Source: CAD feature listing. Evaluate the final solid. Frame: model axes, mm. Face numbers are marked on the shaded views. A direction names the side the tool comes from. Coordinates: 2 decimals unless noted, no trailing zeros. Loops run counter-clockwise (first coordinate to the right, second up) from the corner with the lowest first, then second, coordinate; pieces in that order, holes last.
Item 1: Section query D-D, the plane x = 27. Return the cut outline in (y, z).
Item 2: Reachability of the marked faces 5, 6 and 7 from +Z, -Z, +X, -X, +Y, -Y: full face, straight path, thin tool, end or side. Return the list, or none.
Item 3: Section query A-A, the plane y = 0. Return the cut outline in (x, z), then the cut area to 3 significant figures.
Item 4: Pull-direction query (Y, two-part tool) for the marked faces 1, 2, 3 and 4; classes: +Y half, -Y half, draft (parallel to the pull), parting line (faces both ways), or undercut.
Item 5: Line query: probe 1 along Y at (x, z) = (32.5, 0.75); probe 2 along X at (y, z) = (2.5, -3). Output: solid intervals per line, ascending.
Item 6: Section query B-B, the plane z = -14.5. Return the cut outline in (x, y), then the cut area to 3 significant figures.
Item 7: Pin query (flat end, axial travel): pin 1 Ø7 at (y, z) = (1, -4) entering from +X; pin 2 Ø10 at (y, z) = (13, -9.5) entering from -X; pin 3 Ø2 at (y, z) = (-11, -13) entering from +X; pin 4 Ø10 at (y, z) = (2.5, -2) entering from -X. Return the tip coordinate at first contact, or that it passes through.
Item 8: Section query C-C, the plane y = 10. Return the cut outline in (x, z).
```python
from build123d import *

# Parameters (mm, degrees)
F0_W             = 75
F0_H             = 35
F1_DEPTH         = 1
F3_DEPTH         = 30
F5_DEPTH         = 35
F6_R             = 5
F7_R             = 1.75
F8_DEPTH         = 25
F9_DEPTH         = 1
F10_DEPTH        = 65.4
F13_DEPTH        = 35.6
F13_COPIES_COUNT = 6
F14_T1_DEPTH     = 16.1153550717
F14_T3_DEPTH     = 16.1153550717
F14_T5_DEPTH     = 16.1153550717
F14_T7_DEPTH     = 16.1153550717
F14_T9_DEPTH     = 16.1153550717
F14_T11_DEPTH    = 16.1153550717
F14_T13_DEPTH    = 16.1153550717
F14_T15_DEPTH    = 16.1153550717
F14_T17_DEPTH    = 16.1153550717
F14_T19_DEPTH    = 16.1153550717


# Not quite as in the source:
# - a fillet or chamfer that OpenCascade refuses, or shapes differently, is made with other operations: its cross-section is extruded or revolved along the edge and cut away or added
# - a pattern or mirror of a feature is missing from the dataset's text; its kind, count and spacing are read off the source's solid


with BuildPart() as f1:
    # F0 (on Top) → F1 (new body)
    with BuildSketch(Plane.XY):
        Rectangle(F0_W, F0_H)
    extrude(amount=F1_DEPTH)

    # F2 (on Top) → F3 (join)
    with BuildSketch(Plane.XY):
        Polygon((24.1481456572, 6.4704761276), (17.6776695297, 17.6776695297), (6.4704761276, 24.1481456572), (-6.4704761276, 24.1481456572), (-17.6776695297, 17.6776695297), (-24.1481456572, 6.4704761276), (-24.1481456572, -6.4704761276), (-17.6776695297, -17.6776695297), (-6.4704761276, -24.1481456572), (6.4704761276, -24.1481456572), (17.6776695297, -17.6776695297), (24.1481456572, -6.4704761276), align=None)
    extrude(amount=-F3_DEPTH)

    # F4 (on face) → F5 (cut)
    with BuildSketch(Plane(origin=(0, 0, -30), x_dir=(1, 0, 0), z_dir=(0, 0, -1))):
        Polygon((6.2116570825, -23.1822198309), (16.9705627485, -16.9705627485), (23.1822198309, -6.2116570825), (23.1822198309, 6.2116570825), (16.9705627485, 16.9705627485), (6.2116570825, 23.1822198309), (-6.2116570825, 23.1822198309), (-16.9705627485, 16.9705627485), (-23.1822198309, 6.2116570825), (-23.1822198309, -6.2116570825), (-16.9705627485, -16.9705627485), (-6.2116570825, -23.1822198309), align=None)
    extrude(amount=-F5_DEPTH, mode=Mode.SUBTRACT)

    # F6
    f6_edges = [f1.edges().sort_by_distance(p)[0] for p in [
        (37.5, -17.5, 0.5),
        (37.5, 17.5, 0.5),
        (-37.5, -17.5, 0.5),
        (-37.5, 17.5, 0.5),
    ]]
    fillet(f6_edges, radius=F6_R)

    # F7 (on Top) → F8 (cut)
    with BuildSketch(Plane.XY):
        with Locations((-32.5, 10)):
            Circle(F7_R)
        with Locations((-32.5, -10)):
            Circle(F7_R)
        with Locations((32.5, -10)):
            Circle(F7_R)
        with Locations((32.5, 10)):
            Circle(F7_R)
    extrude(amount=F8_DEPTH, mode=Mode.SUBTRACT)

    # F2 (on Top) → F9 (join)
    with BuildSketch(Plane.XY):
        Polygon((24.1481456572, 6.4704761276), (17.6776695297, 17.6776695297), (6.4704761276, 24.1481456572), (-6.4704761276, 24.1481456572), (-17.6776695297, 17.6776695297), (-24.1481456572, 6.4704761276), (-24.1481456572, -6.4704761276), (-17.6776695297, -17.6776695297), (-6.4704761276, -24.1481456572), (6.4704761276, -24.1481456572), (17.6776695297, -17.6776695297), (24.1481456572, -6.4704761276), align=None)
    extrude(amount=F9_DEPTH)

    # F4 (on face) → F10 (cut)
    with BuildSketch(Plane(origin=(0, 0, -30), x_dir=(1, 0, 0), z_dir=(0, 0, -1))):
        Polygon((6.2116570825, -23.1822198309), (16.9705627485, -16.9705627485), (23.1822198309, -6.2116570825), (23.1822198309, 6.2116570825), (16.9705627485, 16.9705627485), (6.2116570825, 23.1822198309), (-6.2116570825, 23.1822198309), (-16.9705627485, 16.9705627485), (-23.1822198309, 6.2116570825), (-23.1822198309, -6.2116570825), (-16.9705627485, -16.9705627485), (-6.2116570825, -23.1822198309), align=None)
    extrude(amount=-F10_DEPTH, mode=Mode.SUBTRACT)

    # F12 (on Right) → F13 (cut)
    with BuildSketch(Plane.YZ):
        with BuildLine():
            ThreePointArc((-8, -13), (0, -21), (8, -13))
            ThreePointArc((8, -13), (0, -5), (-8, -13))
        make_face()
        with BuildLine():
            Line((8, -37.0977148414), (8, -13))
            ThreePointArc((8, -13), (0, -21), (-8, -13))
            Line((-8, -13), (-8, -36.2910553813))
            Line((-8, -36.2910553813), (8, -37.0977148414))
        make_face()
    f13 = extrude(amount=F13_DEPTH, mode=Mode.SUBTRACT)

    # F13_copies: F13 ×6 about axis
    f13_copies_axis = Axis((0, 0, 0), (0, 0, 1))
    for i in range(1, F13_COPIES_COUNT):
        add(f13.rotate(f13_copies_axis, i * 360 / F13_COPIES_COUNT), mode=Mode.SUBTRACT)

    # F14: fillet of radius 3 on 12 edges, made by hand

    # F14_s2 → F14_t1 (cut)
    with BuildSketch(Plane.YZ.offset(14.6497195661)):
        with BuildLine():
            ThreePointArc((-11, -30), (-8.8786796564, -29.1213203436), (-8, -27))
            Line((-8, -27), (-8, -30))
            Line((-8, -30), (-11, -30))
        make_face()
        with BuildLine():
            ThreePointArc((8, -27), (8.8786796564, -29.1213203436), (11, -30))
            Line((11, -30), (8, -30))
            Line((8, -30), (8, -27))
        make_face()
    extrude(amount=F14_T1_DEPTH, mode=Mode.SUBTRACT)

    # F14_s4 → F14_t3 (cut)
    with BuildSketch(Plane.YZ.offset(-30.7650746377)):
        with BuildLine():
            ThreePointArc((-8, -27), (-8.8786796564, -29.1213203436), (-11, -30))
            Line((-11, -30), (-8, -30))
            Line((-8, -30), (-8, -27))
        make_face()
        with BuildLine():
            ThreePointArc((8, -27), (8.8786796564, -29.1213203436), (11, -30))
            Line((11, -30), (8, -30))
            Line((8, -30), (8, -27))
        make_face()
    extrude(amount=F14_T3_DEPTH, mode=Mode.SUBTRACT)

    # F14_s6 → F14_t5 (cut)
    with BuildSketch(Plane(origin=(-15.3825373189, -26.6433361856, 0), x_dir=(0, 0, 1), z_dir=(0.5, 0.8660254038, 0))):
        with BuildLine():
            ThreePointArc((-30, -11), (-29.1213203436, -8.8786796564), (-27, -8))
            Line((-27, -8), (-30, -8))
            Line((-30, -8), (-30, -11))
        make_face()
    extrude(amount=F14_T5_DEPTH, mode=Mode.SUBTRACT)

    # F14_s8 → F14_t7 (cut)
    with BuildSketch(Plane(origin=(-7.324859783, 12.6870293026, 0), x_dir=(0, 0, 1), z_dir=(-0.5, 0.8660254038, 0))):
        with BuildLine():
            ThreePointArc((-30, -11), (-29.1213203436, -8.8786796564), (-27, -8))
            Line((-27, -8), (-30, -8))
            Line((-30, -8), (-30, -11))
        make_face()
    extrude(amount=F14_T7_DEPTH, mode=Mode.SUBTRACT)

    # F14_s10 → F14_t9 (cut)
    with BuildSketch(Plane(origin=(-7.324859783, -12.6870293026, 0), x_dir=(0, 0, 1), z_dir=(-0.5, -0.8660254038, 0))):
        with BuildLine():
            ThreePointArc((-27, -8), (-29.1213203436, -8.8786796564), (-30, -11))
            Line((-30, -11), (-30, -8))
            Line((-30, -8), (-27, -8))
        make_face()
    extrude(amount=F14_T9_DEPTH, mode=Mode.SUBTRACT)

    # F14_s12 → F14_t11 (cut)
    with BuildSketch(Plane(origin=(7.324859783, 12.6870293026, 0), x_dir=(0, 0, 1), z_dir=(0.5, 0.8660254038, 0))):
        with BuildLine():
            ThreePointArc((-27, -8), (-29.1213203436, -8.8786796564), (-30, -11))
            Line((-30, -11), (-30, -8))
            Line((-30, -8), (-27, -8))
        make_face()
    extrude(amount=F14_T11_DEPTH, mode=Mode.SUBTRACT)

    # F14_s14 → F14_t13 (cut)
    with BuildSketch(Plane(origin=(-15.3825373189, 26.6433361856, 0), x_dir=(0, 0, 1), z_dir=(0.5, -0.8660254038, 0))):
        with BuildLine():
            ThreePointArc((-30, -11), (-29.1213203436, -8.8786796564), (-27, -8))
            Line((-27, -8), (-30, -8))
            Line((-30, -8), (-30, -11))
        make_face()
    extrude(amount=F14_T13_DEPTH, mode=Mode.SUBTRACT)

    # F14_s16 → F14_t15 (cut)
    with BuildSketch(Plane(origin=(15.3825373189, -26.6433361856, 0), x_dir=(0, 0, 1), z_dir=(-0.5, 0.8660254038, 0))):
        with BuildLine():
            ThreePointArc((-30, -11), (-29.1213203436, -8.8786796564), (-27, -8))
            Line((-27, -8), (-30, -8))
            Line((-30, -8), (-30, -11))
        make_face()
    extrude(amount=F14_T15_DEPTH, mode=Mode.SUBTRACT)

    # F14_s18 → F14_t17 (cut)
    with BuildSketch(Plane(origin=(15.3825373189, 26.6433361856, 0), x_dir=(0, 0, 1), z_dir=(-0.5, -0.8660254038, 0))):
        with BuildLine():
            ThreePointArc((-30, -11), (-29.1213203436, -8.8786796564), (-27, -8))
            Line((-27, -8), (-30, -8))
            Line((-30, -8), (-30, -11))
        make_face()
    extrude(amount=F14_T17_DEPTH, mode=Mode.SUBTRACT)

    # F14_s20 → F14_t19 (cut)
    with BuildSketch(Plane(origin=(7.324859783, -12.6870293026, 0), x_dir=(0, 0, 1), z_dir=(0.5, -0.8660254038, 0))):
        with BuildLine():
            ThreePointArc((-27, -8), (-29.1213203436, -8.8786796564), (-30, -11))
            Line((-30, -11), (-30, -8))
            Line((-30, -8), (-27, -8))
        make_face()
    extrude(amount=F14_T19_DEPTH, mode=Mode.SUBTRACT)


solid = f1.part
```
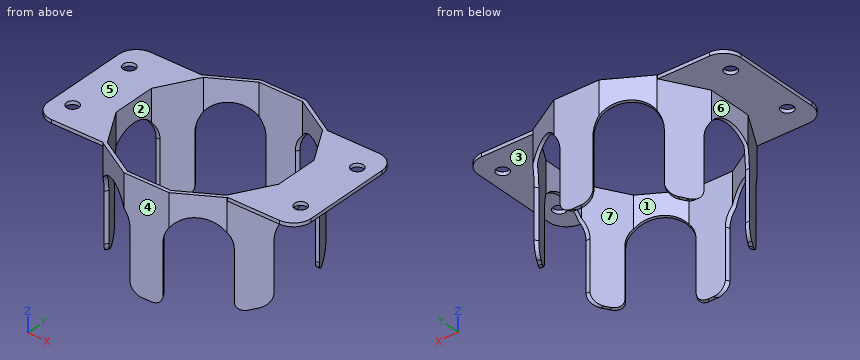
Verdict:
1. outline: (-17.5, 0) - (17.5, 0) - (17.5, 1) - (-17.5, 1) - close
2. face 5: +Z, +X, -X, +Y, -Y
2. face 6: -Z, -X, +Y, -Y
2. face 7: +Z, -Z
3. outline: (-37.5, 0) - (-24.15, 0) - (-24.15, -5) - (-23.18, -5) - (-23.18, 1) - (-37.5, 1) - close; (23.18, -5) - (24.15, -5) - (24.15, 0) - (37.5, 0) - (37.5, 1) - (23.18, 1) - close
3. area: 38.3 mm2
4. face 1: undercut
4. face 2: undercut
4. face 3: draft
4. face 4: -Y half
5. probe 1: y = -17.5 to -11.75, -8.25 to 8.25, 11.75 to 17.5
5. probe 2: x = -24.15 to -23.18, 23.18 to 24.15
6. outline: (-23.27, -8) - (-18.56, -16.15) - (-18, -15.18) - (-22.15, -8) - close; (-23.27, 8) - (-22.15, 8) - (-18, 15.18) - (-18.56, 16.15) - close; (-4.7, -24.15) - (4.7, -24.15) - (4.15, -23.18) - (-4.15, -23.18) - close; (-4.7, 24.15) - (-4.15, 23.18) - (4.15, 23.18) - (4.7, 24.15) - close; (18, -15.18) - (18.56, -16.15) - (23.27, -8) - (22.15, -8) - close; (18, 15.18) - (22.15, 8) - (23.27, 8) - (18.56, 16.15) - close
6. area: 51.3 mm2
7. pin 1: stops at x = 24.15
7. pin 2: stops at x = -23.27
7. pin 3: stops at x = 22.11
7. pin 4: stops at x = -37.5
8. outline: (-37.5, 0) - (-34.25, 0) - (-34.25, 1) - (-37.5, 1) - close; (-30.75, 0) - (-22.11, 0) - (-22.11, -29.83) - (-21, -29.83) - (-21, 1) - (-30.75, 1) - close; (21, -29.83) - (22.11, -29.83) - (22.11, 0) - (30.75, 0) - (30.75, 1) - (21, 1) - close; (34.25, 0) - (37.5, 0) - (37.5, 1) - (34.25, 1) - close
